Can you work these out from the model? Positions are in its coordinate system, mm. Give positions to 0.01 mm unless a question says otherwise; leave off trailing zeros. Loops run counter-clockwise (first coordinate to the right, second up) from the corner with the lowest first, then second, coordinate; pieces in that order, holes last. Notation, with made-up numbers: (30.5, 13.25) - (64.5, 13.25) arc R22 cw to (64.5, 29.25) - close; hole circle Ø6 at (86.25, 0.5). An arc over 180 degrees is marked (long way). Answer as a JSON object with one key per item and string values. Group by question number.
Item 1: Suppose I cut it at D-D on x = -72. Write out the boundary of the cut face in (y, z), and give its area (3 significant figures).
Item 2: Suppose I cut it at B-B on z = 0.6. Write out the boundary of the cut face in (x, y), and give its area (3 significant figures).
Item 3: Suppose I cut it at A-A on y = -6.5. Write out the boundary of the cut face in (x, z).
Item 4: Will these pins go through, and if not, where does the flat tip stop? pin 1 (0.9 mm diameter, centred on x = 74, z = 1.5, fed in from +Y); pin 2 (6 mm diameter, centred on x = 80, y = -6.5, fed in from +Z); pin 3 (0.9 mm diameter, centred on y = 17.5, z = 1, fed in from +X); pin 4 (0.9 mm diameter, centred on y = -26.5, z = 2, fed in from -X).
Item 5: Please list where these lines run through material, in increasing order: L1, parallel to Y at x = 80, z = 2.05; L2, parallel to Y at x = -76.5, z = 0.6; L3, parallel to X at y = -0.5, z = 1.35.
Autodesk Inventor part; units mm, degrees
ref_plane "YZ Plane" through (0, 0, 0) normal (1, 0, 0) x (0, 1, 0)
ref_plane "XZ Plane" through (0, 0, 0) normal (0, 1, 0) x (-1, 0, 0)
ref_plane "XY Plane" through (0, 0, 0) normal (0, 0, 1) x (1, 0, 0)
sketch "Sketch1" plane through (0, 0, 0) normal (0, 0, 1) x (1, 0, 0)
  line L0 (0, 44.1) -> (0, -44.1) construction
  line L1 (-4897.1485, 0) -> (4897.1485, 0) construction
  line L2 (0, -31.5) -> (-68, -31.5)
  line L3 (-68, -31.5) -> (-68, -18)
  line L4 (-68, -18) -> (-80, -18)
  line L5 (-85, 0) -> (-85, -22.0738) construction
  line L6 (-75, -22.5739) -> (-75, 22.5739) construction
  circle A0 centre (-80, -13) radius 2.5
  circle A1 centre (-80, 0) radius 2.5
  line L7 (-80, 0) -> (-80, -13) construction
  arc A2 (-81.8558, -8.3571) -> (-80, -18) centre (-80, -13) ccw
  arc A3 (-85, 0) -> (-81.8558, -4.6429) centre (-80, 0) ccw
  arc A4 (-81.8558, -8.3571) -> (-81.8558, -4.6429) centre (-82.5981, -6.5) ccw
  line L8 (0, 31.5) -> (-68, 31.5)
  line L9 (-68, 31.5) -> (-68, 18)
  line L10 (-68, 18) -> (-80, 18)
  line L11 (-85, 0) -> (-85, 22.0738) construction
  line L12 (-75, 22.5739) -> (-75, -22.5739) construction
  circle A5 centre (-80, 13) radius 2.5
  circle A6 centre (-80, 0) radius 2.5
  line L13 (-80, 0) -> (-80, 13) construction
  arc A7 (-80, 18) -> (-81.8558, 8.3571) centre (-80, 13) ccw
  arc A8 (-81.8558, 4.6429) -> (-85, 0) centre (-80, 0) ccw
  arc A9 (-81.8558, 4.6429) -> (-81.8558, 8.3571) centre (-82.5981, 6.5) ccw
  line L14 (4897.1485, 0) -> (-4897.1485, 0) construction
  line L15 (0, -31.5) -> (68, -31.5)
  line L16 (68, -31.5) -> (68, -11.5)
  line L17 (68, -11.5) -> (80, -11.5)
  line L18 (68, 11.5) -> (80, 11.5)
  line L19 (68, 31.5) -> (68, 11.5)
  line L20 (0, 31.5) -> (68, 31.5)
  line L21 (80, 11.5) -> (80, -11.5) construction
  circle A10 centre (80, -6.5) radius 2.5
  circle A11 centre (80, 6.5) radius 2.5
  line L22 (75, 22.5739) -> (75, -22.5739) construction
  line L23 (75, 22.5739) -> (75, -22.5739) construction
  arc A12 (80, -11.5) -> (81.8558, -1.8571) centre (80, -6.5) ccw
  arc A13 (81.8558, 1.8571) -> (80, 11.5) centre (80, 6.5) ccw
  arc A14 (81.8558, 1.8571) -> (81.8558, -1.8571) centre (82.5981, 0) ccw
  point P0 (0, 0)
  dimension "d0" = 31.5
  dimension "d2" = 7
  dimension "d4" = 5
  dimension "d5" = 5
  dimension "d6" = 5
  dimension "d7" = 5
  dimension "d8" = 13
  dimension "d9" = 5
  dimension "d10" = 2
  dimension "d11" = 2.5
  dimension "d12" = 5
  dimension "d13" = 2.5
  dimension "d14" = 5
  dimension "d15" = 13
  dimension "d16" = 2
extrude "Extrusion1" add sketch "Sketch1" along normal blind 3
equation "\"d0\" = 0.5 * PowerPCB_Width"
equation "\"d2\" = Interface_Thickness"
equation "\"d7\" = d6"
equation "\"d12\" = d4"
equation "\"d13\" = d11"
equation "\"d14\" = d9"
equation "\"d17\" = PowerPCB_Thickness"
equation "\"Heatsink_Thickness\" = 5"
equation "\"Heatsink_Width\" = 65"
equation "\"Cover_Thickness\" = 2"
equation "\"PowerPCB_Minus_Height\" = 1.2"
equation "\"PowerPCB_Width\" = 63"
equation "\"Interface_Thickness\" = 7"
equation "\"PowerPCB_Thickness\" = 3"
equation "\"PowerPCB_Plus_Height\" = 8"
equation "\"LogicPCB_Width\" = 55"
equation "\"LogicPCB_Thickness\" = 2"
equation "\"LogicPCB_Plus_Height\" = 8"
equation "\"HostPCB_Thickness\" = 1.2"
equation "\"HostPCB_Plus_Height\" = 8"
properties part number "PowerPCB" material "GFRC"
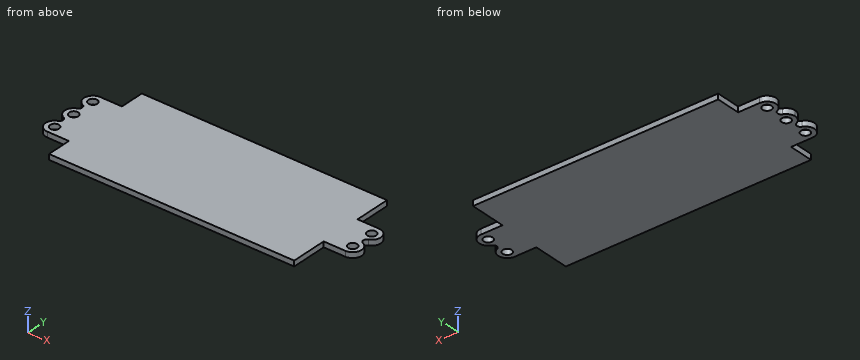
Worked out:
{
 "1": {"outline": "(-18, 0) - (18, 0) - (18, 3) - (-18, 3) - close", "area": "108 mm2"},
 "2": {"outline": "(-85, 0) arc R5 ccw to (-81.86, -4.64) arc R2 cw to (-81.86, -8.36) arc R5 ccw to (-80, -18) - (-68, -18) - (-68, -31.5) - (68, -31.5) - (68, -11.5) - (80, -11.5) arc R5 ccw to (81.86, -1.86) arc R2 cw to (81.86, 1.86) arc R5 ccw to (80, 11.5) - (68, 11.5) - (68, 31.5) - (-68, 31.5) - (-68, 18) - (-80, 18) arc R5 ccw to (-81.86, 8.36) arc R2 cw to (-81.86, 4.64) arc R5 ccw to start; hole circle Ø5 at (-80, -13); hole circle Ø5 at (-80, 0); hole circle Ø5 at (-80, 13); hole circle Ø5 at (80, -6.5); hole circle Ø5 at (80, 6.5)", "area": "9,380 mm2"},
 "3": {"outline": "(-80.6, 0) - (77.5, 0) - (77.5, 3) - (-80.6, 3) - close; (82.5, 0) - (85, 0) - (85, 3) - (82.5, 3) - close"},
 "4": {"pin 1": "stops at y = 11.5", "pin 2": "stops at z = 3", "pin 3": "stops at x = 68", "pin 4": "stops at x = -68"},
 "5": {"L1": "y = -11.5 to -9, -4 to 4, 9 to 11.5", "L2": "y = -18 to 18", "L3": "x = -84.97 to -82.45, -77.55 to 80.66"}
}
